Read the model definition and answer for the solid it produces. Units are mm, in the model's axes. A direction names the side the tool comes from. Coordinates: 2 decimals unless noted, no trailing zeros. Loops run counter-clockwise (first coordinate to the right, second up) from the corner with the lowest first, then second, coordinate; pieces in that order, holes last.
Q1. Section C-C (z = 6.5) is taken. Give the vertices of the cut face in (x, y).
Q2. Section B-B (x = 65) is taken. Give the vertices of the cut face in (y, z).
Q3. Which of the six approach directions +Z, -Z, +X, -X, +Y, -Y give full straight-line access (tool end or side, diameter ignored) to faces 1 (the face through (-255.713, -2.176, -8.623)), 2 (the face through (140, 1, -8))?
Q4. Straight lines are drawn through the part: line 1 (Y direction, x = 19.5, z = 9); line 2 (X direction, y = -9, z = -6.5). For each, find the intervals that lie inside material, in ascending order.
Q5. Section A-A (y = -3) is taken. Give the vertices of the cut face in (x, z), then the cut area to 3 significant figures.
Q6. Flat-ended cylindrical pins translate along their axes: P1, Ø4, axis at x = -4, z = -7.5, coming from the +Y side; P2, Ø9, axis at x = 131.5, y = -2.5, coming from the +Z side. Find the tip coordinate at first contact, or state that the pin passes through.
from build123d import *

# Parameters (mm, degrees)
BOSS_EXTRUDE1_DEPTH = 270
CUT_EXTRUDE1_DEPTH  = 271.370116692
CUT_EXTRUDE2_DEPTH  = 262.462086162


with BuildPart() as part:
    # Sketch1 → Boss-Extrude1 (new, symmetric)
    with BuildSketch(Plane(origin=(0, 0, 0), x_dir=(0, 0, -1), z_dir=(1, 0, 0))):
        Polygon((8, 10), (10, 10), (10, -10), (-10, -10), (-10, -8), (8, -8), align=None)
    extrude(amount=BOSS_EXTRUDE1_DEPTH, both=True)

    # Sketch2 → Cut-Extrude1 (cut, symmetric)
    with BuildSketch(Plane(origin=(0, 0, 0), x_dir=(1, 0, 0), z_dir=(0, 1, 0))):
        with BuildLine():
            Line((248.65, 2.75), (250.65, 2.75))
            ThreePointArc((250.65, 2.75), (253.4, 0), (250.65, -2.75))
            Line((250.65, -2.75), (248.65, -2.75))
            ThreePointArc((248.65, -2.75), (245.9, 0), (248.65, 2.75))
        make_face()
        with BuildLine():
            ThreePointArc((250.65, -10), (260.65, 0), (250.65, 10))
            Line((250.65, 10), (270, 10))
            Line((270, 10), (270, -10))
            Line((270, -10), (250.65, -10))
        make_face()
    cut_extrude1 = extrude(amount=CUT_EXTRUDE1_DEPTH, both=True, mode=Mode.SUBTRACT)

    # Mirror1: Cut-Extrude1 across plane
    add(cut_extrude1.mirror(Plane(origin=(0, 0, 0), x_dir=(0, 0, 1), z_dir=(1, 0, 0))), mode=Mode.SUBTRACT)

    # Sketch3 → Cut-Extrude2 (cut, through all)
    with BuildSketch(Plane.XY.offset(-8)):
        Polygon((-20, -8), (20, -8), (22.706021628, 10), (-22.706021628, 10), align=None)
    extrude(amount=-CUT_EXTRUDE2_DEPTH, mode=Mode.SUBTRACT)


solid = part.part
Numbers:
1. outline: (-258.25, -10) - (258.25, -10) - (258.25, -8) - (-258.25, -8) - close
2. outline: (-10, -10) - (10, -10) - (10, -8) - (-8, -8) - (-8, 10) - (-10, 10) - close
3. face 1: -X, +Y, -Y
3. face 2: +Z, +X, -X, +Y
4. line 1: y = -10 to -8
4. line 2: x = -258.25 to 258.25
5. outline: (-256.65, -8) arc R10 ccw to (-250.65, -10) - (-20.75, -10) - (-20.75, -8) - close; (20.75, -10) - (250.65, -10) arc R10 ccw to (256.65, -8) - (20.75, -8) - close
5. area: 936 mm2
6. P1: stops at y = -8
6. P2: stops at z = -8
